For this review, take the finished solid that the model builds, in its own axes (mm). Face numbers are marked on the shaded views. A direction names the side the tool comes from. Round coordinates to 2 decimals unless told otherwise and drop trailing zeros. Write each loop counter-clockwise with the first axis right and the second up, starting at its lowest first coordinate (ties: lowest second). Pieces come first, ordered by that corner, then holes. Notation, with made-up numbers: M -38.75,20.25 L 16.25,20.25 A26 ccw 16.25,48.25 Z; hole C 41,2.25 d7. An arc over 180 degrees is marked long. Answer in a Markdown table with one row per item.
Autodesk Inventor part; units mm, degrees
ref_plane "YZ Plane" through (0, 0, 0) normal (1, 0, 0) x (0, 1, 0)
ref_plane "XZ Plane" through (0, 0, 0) normal (0, 1, 0) x (-1, 0, 0)
ref_plane "XY Plane" through (0, 0, 0) normal (0, 0, 1) x (1, 0, 0)
sketch "Sketch1" plane through (0, 0, 0) normal (0, 0, 1) x (1, 0, 0)
  circle A0 centre (109.5845, 54.716) radius 3.175 construction
  line L0 (765.556, 95.25) -> (765.556, -44.45) construction
  line L1 (0, 95.25) -> (765.556, 95.25) construction
  line L2 (0, -44.45) -> (0, 95.25) construction
  line L3 (765.556, -44.45) -> (0, -44.45) construction
  arc A1 (100.6141, 53.9869) -> (110.3117, 45.7454) centre (109.5836, 54.7149) ccw
  line L4 (123.1622, 19.6987) -> (119.3655, 66.4721)
  circle A2 centre (109.5836, 54.7149) radius 8.999
  circle A3 centre (109.5845, 54.716) radius 6
  circle A4 centre (109.5845, 54.716) radius 6.254
  circle A5 centre (109.5845, 54.716) radius 3.3
  point P0 (0, 0)
  dimension "d0" = 0.254
  dimension "d1" = 6.6
extrude "Extrusion1" add sketch "Sketch1" along normal blind 7.1882 contours A2 A1 | A3 | A4
sketch "Sketch2" plane through (109.5836, 54.7149, 7.1882) normal (0, 0, 1) x (1, 0, 0)
  circle A0 centre (0.0009, 0.0011) radius 3.3
  line L0 (-4.9991, 2.8878) -> (0.0009, 5.7746)
  line L1 (0.0009, 5.7746) -> (5.0009, 2.8878)
  line L2 (5.0009, 2.8878) -> (5.0009, -2.8857)
  line L3 (5.0009, -2.8857) -> (0.0009, -5.7724)
  line L4 (0.0009, -5.7724) -> (-4.9991, -2.8857)
  line L5 (-4.9991, -2.8857) -> (-4.9991, 2.8878)
  line L6 (0.0009, 6.0679) -> (-5.2531, 3.0345)
  line L7 (-5.2531, 3.0345) -> (-5.2531, -3.0323)
  line L8 (-5.2531, -3.0323) -> (0.0009, -6.0657)
  line L9 (0.0009, -6.0657) -> (5.2549, -3.0323)
  line L10 (5.2549, -3.0323) -> (5.2549, 3.0345)
  line L11 (5.2549, 3.0345) -> (0.0009, 6.0679)
  circle A1 centre (0, 0) radius 8.999
  point P0 (-109.5836, -54.7149)
  point P1 (-4.9991, -2.8857)
  dimension "d4" = 0.254
extrude "Extrusion2" add sketch "Sketch2" along normal blind 6.0198 contours A1
fillet "Fillet1" radius 0.635 6 edges at (104.3305, 54.716, 13.208) (106.9575, 50.1659, 13.208) (112.2115, 50.1659, 13.208) (114.8385, 54.716, 13.208) (112.2115, 59.2661, 13.208) (106.9575, 59.2661, 13.208)
properties part number "ActuatorSpacer"
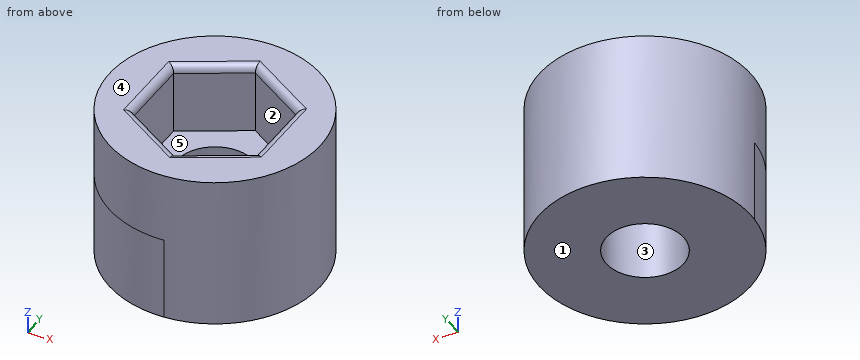
Q1. Take a section at C-C (x = 102.75). State the section outline as (y, z) points.
Found:
| item | result |
|---|---|
| outline | M 48.86,0 L 60.57,0 L 60.57,13.21 L 48.86,13.21 Z |
Q2. For probe 1 along X at (y, z) = (54.75, 2.5); probe 2 along Y at (x, z) = (111.75, 3.5); probe 3 along Y at (x, z) = (108.5, 5.25), list the stretches that pass through material, from the lowest coordinate up.
Found:
| item | result |
|---|---|
| probe 1 | 100.58 to 106.28, 112.88 to 118.58 |
| probe 2 | 45.98 to 52.23, 57.21 to 63.45 |
| probe 3 | 45.78 to 51.6, 57.83 to 63.65 |
Q3. Mouldability with a two-part tool opening along Y and no side actions: class the marked faces 3, 4 and 5 as +Y half, -Y half, draft (parallel to the pull), parting line (faces both ways), or undercut.
Found:
| item | result |
|---|---|
| face 3 | undercut |
| face 4 | draft |
| face 5 | undercut |
Q4. Machinability: for the marked faces 1 and 2, which of the approach directions +Z, -Z, +X, -X, +Y, -Y give a long, thin tool a straight path to every point of the face, cutting with its end or side? Answer none if there is none.
Found:
| item | result |
|---|---|
| face 1 | -Z, +X, -X, +Y, -Y |
| face 2 | +Z |
Q5. Take a section at A-A (y = 55). State the section outline as (x, z) points (1 decimal), then the cut area to 3 significant figures.
Found:
| item | result |
|---|---|
| outline | M 100.6,0 L 106.3,0 L 106.3,7.2 L 104.3,7.2 L 104.3,12.6 A0.6 ccw 103.7,13.2 L 100.6,13.2 Z; M 112.9,0 L 118.6,0 L 118.6,13.2 L 115.5,13.2 A0.6 ccw 114.8,12.6 L 114.8,7.2 L 112.9,7.2 Z |
| area | 127 mm² |
Q6. Insertion check: P1, Ø3, axis at x = 106, y = 53, coming from the -Z side; P2, Ø2, axis at y = 48, z = 3.5, coming from the -X side; P3, Ø3, axis at y = 50.5, z = 6.5, coming from the +X side; P4, Ø2, axis at x = 102.5, z = 10, coming from the -Y side. Each pin has a flat end and moves straight along its axis. Give the tip position at first contact, or say it passes through.
Found:
| item | result |
|---|---|
| P1 | z = 0 |
| P2 | x = 102.63 |
| P3 | x = 118.16 |
| P4 | y = 48.08 |
Q7. Take a section at B-B (z = 10.5). State the section outline as (x, y) points.
Found:
| item | result |
|---|---|
| outline | C 109.58,54.71 d18; hole M 104.33,51.68 L 109.58,48.65 L 114.84,51.68 L 114.84,57.75 L 109.58,60.78 L 104.33,57.75 Z |
Q8. Take a section at D-D (y = 62). State the section outline as (x, z) points.
Found:
| item | result |
|---|---|
| outline | M 104.3,0 L 114.87,0 L 114.87,13.21 L 104.3,13.21 Z |
